Drawing for the job (mm, zero at the part's lowest x, y, z). Give positions to 0.01 mm unless a question says otherwise; leave off trailing zeros. Order: outer loops, then holes, each group sorted by start corner. A loop starts at its lowest first (then second) coordinate and runs counter-clockwise, first axis right, second up. Notation, with made-up numbers: (-31.5, -12.75) - (17.5, -12.75) arc R24 cw to (17.5, 21.25) - close; hole circle Ø5 at (-10.75, 48.25). An arc over 180 degrees is marked (long way). One line per item, written item: value.
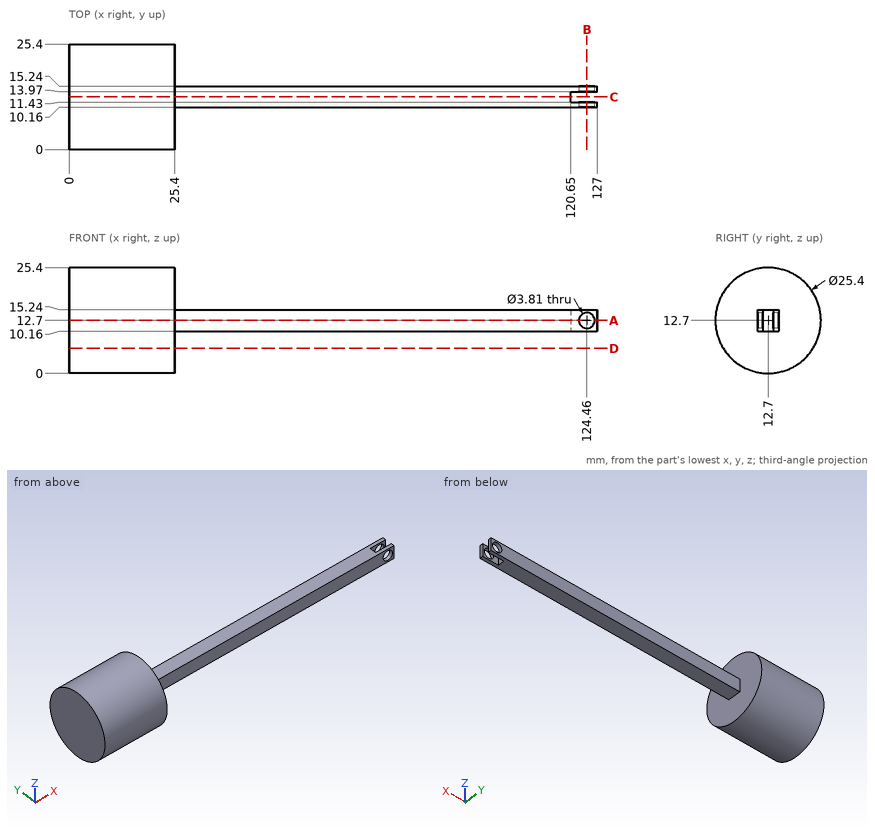
1) Cut at C-C, the plane y = 12.7. Give the cut face in (x, z).
Outcome:
outline: (0, 0) - (25.4, 0) - (25.4, 10.16) - (120.65, 10.16) - (120.65, 15.24) - (25.4, 15.24) - (25.4, 25.4) - (0, 25.4) - close
2) Cut at B-B, the plane x = 124.46. Give the cut face in (y, z) (3 decimals), then the cut area to 3 significant figures.
Outcome:
outline: (10.16, 10.16) - (11.43, 10.16) - (11.43, 10.795) - (10.16, 10.795) - close; (10.16, 14.605) - (11.43, 14.605) - (11.43, 15.24) - (10.16, 15.24) - close; (13.97, 10.16) - (15.24, 10.16) - (15.24, 10.795) - (13.97, 10.795) - close; (13.97, 14.605) - (15.24, 14.605) - (15.24, 15.24) - (13.97, 15.24) - close
area: 3.23 mm^2
3) Cut at A-A, the plane z = 12.7. Give the cut face in (x, y) (3 decimals), then the cut area to 3 significant figures.
Outcome:
outline: (0, 0) - (25.4, 0) - (25.4, 10.16) - (122.555, 10.16) - (122.555, 11.43) - (120.65, 11.43) - (120.65, 13.97) - (122.555, 13.97) - (122.555, 15.24) - (25.4, 15.24) - (25.4, 25.4) - (0, 25.4) - close; (126.365, 10.16) - (127, 10.16) - (127, 11.43) - (126.365, 11.43) - close; (126.365, 13.97) - (127, 13.97) - (127, 15.24) - (126.365, 15.24) - close
area: 1,140 mm^2
4) Cut at D-D, the plane z = 6. Give the cut face in (x, y).
Outcome:
outline: (0, 1.91) - (25.4, 1.91) - (25.4, 23.49) - (0, 23.49) - close
5) Pin check, flat tips, straight feed: pin 1 (5.5 mm diameter, centred on x = 56.5, y = 11.5, fed in from -Z); pin 2 (5.5 mm diameter, centred on x = 71, z = 13.5, fed in from +Y); pin 3 (6 mm diameter, centred on x = 124.46, z = 12.7, fed in from -Y). Stop position of each tip, or through.
Outcome:
pin 1: stops at z = 10.16
pin 2: stops at y = 15.24
pin 3: stops at y = 10.16
6) Drill centre lines: line 1 along Z through (x, y) = (124.46, 14.75) (3 decimals); line 2 along X through (y, z) = (8.25, 5.75); line 3 along Y through (x, z) = (99, 11.25). Where is each one in solid material? Low to high. Write a range as from..to.
Outcome:
line 1: z = 10.16..10.795, 14.605..15.24
line 2: x = 0..25.4
line 3: y = 10.16..15.24
